Study the drawing (mm; zero at the part's minimum x, y, z) and answer. A direction names the side the tool comes from. Coordinates: 2 decimals unless noted, no trailing zeros. Order: outer loops, then holes, each group sorted by start corner. A loop starts at its lowest first (then second) coordinate and runs counter-clockwise, first axis right, second up. Notation, with made-up numbers: (68, 53.25) -> (102, 53.25) arc R30 cw to (102, 80.25) -> close; hole circle Ø2 at (33.5, 24). An arc over 180 degrees is marked (long way). Put each result on its own line as item: value. Start each with the question number.
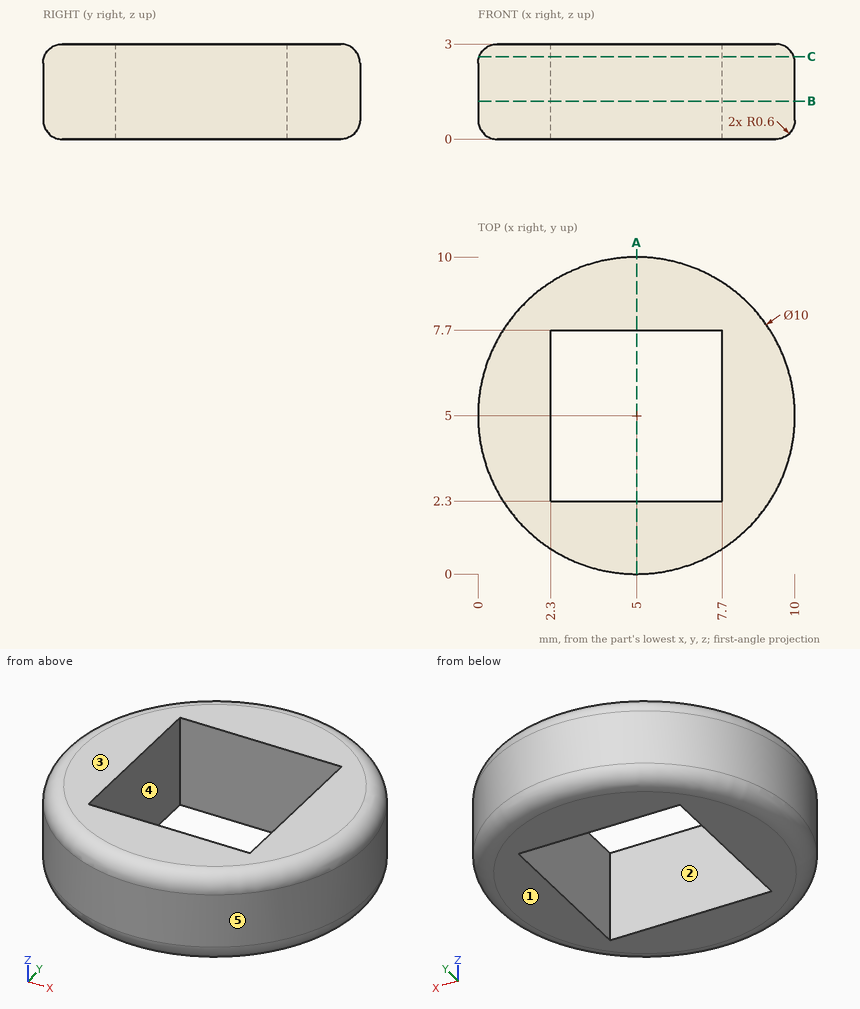
(1) The part is cut by section A-A on x = 5. Determine the outline of the cut face in (y, z), plus the area to 3 significant figures.
(2) Find the intervals of material crossed by L1, parallel to X at y = 6, z = 0.6; L2, parallel to X at y = 6.25, z = 1.45; L3, parallel to Y at x = 5.25, z = 2.35, in increasing order.
(3) The part is cut by section C-C on z = 2.6. Determine the outline of the cut face in (x, y).
(4) For a pull along Y with two mould halves and no side action, classify the marked faces 3, 4 and 5 as released by +Y, released by -Y, zero draft, split by the parting line, or undercut.
(5) A tool of negligible diameter and unlimited length cuts with its end or side. For the marked faces 1 and 2, from which of +Z, -Z, +X, -X, +Y, -Y can it reach the whole face along a straight path? Write none if from no direction.
(6) The part is cut by section B-B on z = 1.2. Determine the outline of the cut face in (x, y), plus the area to 3 significant figures.
(7) This flat-tipped pin is pushed along its axis until it touches: P1, Ø1.5, axis at x = 5.5, y = 4.5, coming from the +Z side. Where does it stop, or does it pass through?
Worked out:
1. outline: (0, 0.6) arc R0.6 ccw to (0.6, 0) -> (2.3, 0) -> (2.3, 3) -> (0.6, 3) arc R0.6 ccw to (0, 2.4) -> close; (7.7, 0) -> (9.4, 0) arc R0.6 ccw to (10, 0.6) -> (10, 2.4) arc R0.6 ccw to (9.4, 3) -> (7.7, 3) -> close
1. area: 13.5 mm2
2. L1: 0.1 to 2.3, 7.7 to 9.9
2. L2: 0.16 to 2.3, 7.7 to 9.84
2. L3: 0.01 to 2.3, 7.7 to 9.99
3. outline: circle Ø9.93 at (5, 5); hole (2.3, 2.3) -> (7.7, 2.3) -> (7.7, 7.7) -> (2.3, 7.7) -> close
4. face 3: zero draft
4. face 4: undercut
4. face 5: split by the parting line
5. face 1: -Z, +X, -X, +Y, -Y
5. face 2: +Z, -Z
6. outline: circle Ø10 at (5, 5); hole (2.3, 2.3) -> (7.7, 2.3) -> (7.7, 7.7) -> (2.3, 7.7) -> close
6. area: 49.4 mm2
7. P1: through
